Geometry: final body of the model. Coordinates: model frame, mm. A direction names the side the tool comes from. Coordinates: 2 decimals unless noted, no trailing zeros. Loops run counter-clockwise (first coordinate to the right, second up) from the corner with the lowest first, then second, coordinate; pieces in that order, holes last. Notation, with made-up numbers: (-23.75, 81.5) - (-14.75, 81.5) arc R33 ccw to (-14.75, 110.5) - close; hole circle Ø4 at (20.25, 62). An arc over 180 degrees is marked (long way). Return JSON: item names as keys, results as strings.
from build123d import *

# Parameters (mm, degrees)
CROQUIS1_W                 = 70
CROQUIS1_H                 = 70
SALIENTE_EXTRUIR1_DEPTH    = 70
CORTAR_EXTRUIR1_DEPTH      = 122.24355653
CORTAR_EXTRUIR1_DEPTH_BACK = 70
CROQUIS3_W                 = 10
CROQUIS3_H                 = 10
CORTAR_EXTRUIR2_DEPTH      = 70
CORTAR_EXTRUIR3_DEPTH      = 122.24355653
CORTAR_EXTRUIR3_DEPTH_BACK = 122.24355653
CORTAR_EXTRUIR4_DEPTH      = 106.44045021
CORTAR_EXTRUIR4_DEPTH_BACK = 106.44045021
CROQUIS5_W                 = 10
CROQUIS5_H                 = 10


with BuildPart() as part:
    # Croquis1 → Saliente-Extruir1 (new body)
    with BuildSketch(Plane(origin=(0, 0, 0), x_dir=(0, 0, -1), z_dir=(1, 0, 0))):
        with Locations((-35, 35)):
            Rectangle(CROQUIS1_W, CROQUIS1_H)
    extrude(amount=SALIENTE_EXTRUIR1_DEPTH)

    # Croquis2 → Cortar-Extruir1 (cut, two sides: drawn at the far end of the back side and taken through both)
    with BuildSketch(Plane.XY.offset(70).offset(-CORTAR_EXTRUIR1_DEPTH_BACK)):
        Polygon((-82.285109819, 188.585089714), (36.299979895, 70), (70, 36.299979895), (188.585089714, -82.285109819), (425.755269142, 154.885069609), (154.885069609, 425.755269142), align=None)
    extrude(amount=CORTAR_EXTRUIR1_DEPTH + CORTAR_EXTRUIR1_DEPTH_BACK, mode=Mode.SUBTRACT)

    # Croquis3 → Cortar-Extruir2 (cut)
    with BuildSketch(Plane(origin=(70, 0, 0), x_dir=(0, 0, -1), z_dir=(1, 0, 0))):
        with Locations((-15, 5)):
            Rectangle(CROQUIS3_W, CROQUIS3_H)
        with Locations((-55, 5)):
            Rectangle(CROQUIS3_W, CROQUIS3_H)
    extrude(amount=-CORTAR_EXTRUIR2_DEPTH, mode=Mode.SUBTRACT)

    # Croquis4 → Cortar-Extruir3 (cut, two sides: drawn at the far end of the back side and taken through both)
    with BuildSketch(Plane.XY.offset(70).offset(-CORTAR_EXTRUIR3_DEPTH_BACK)):
        Polygon((36.299979895, 237.704642169), (36.299979895, 70), (36.299979895, 60), (46.299979895, 60), (214.004622064, 60), (451.174801491, 297.170179428), (273.470159323, 474.874821596), align=None)
    extrude(amount=CORTAR_EXTRUIR3_DEPTH + CORTAR_EXTRUIR3_DEPTH_BACK, mode=Mode.SUBTRACT)

    # Croquis5 → Cortar-Extruir4 (cut, two sides: drawn at the far end of the back side and taken through both)
    with BuildSketch(Plane(origin=(36.299979895, 0, 0), x_dir=(0, 0, -1), z_dir=(1, 0, 0)).offset(-CORTAR_EXTRUIR4_DEPTH_BACK)):
        with Locations((-35, 65)):
            Rectangle(CROQUIS5_W, CROQUIS5_H)
    extrude(amount=CORTAR_EXTRUIR4_DEPTH + CORTAR_EXTRUIR4_DEPTH_BACK, mode=Mode.SUBTRACT)


solid = part.part
Item 1: Section query D-D, the plane z = 58. Return loops of the section in (x, y).
Worked out:
{"outline": "(0, 10) - (70, 10) - (70, 36.3) - (46.3, 60) - (36.3, 60) - (36.3, 70) - (0, 70) - close"}
Item 2: Section query B-B, the plane z = 21.5. Return loops of the section in (x, y), and give its area (3 significant figures).
Worked out:
{"outline": "(0, 0) - (70, 0) - (70, 36.3) - (46.3, 60) - (36.3, 60) - (36.3, 70) - (0, 70) - close", "area": "4,280 mm^2"}
Item 3: Mould query, pull axis Z, two halves, no side actions, for faces 4 (the face through (18, 65, 30)), 5 (the face through (18, 70, 55)), 6 (the face through (35, 35, 70)). Classes: +Z half, -Z half, draft (parallel to the pull), parting line (faces both ways), or undercut.
Worked out:
{"face 4": "undercut", "face 5": "draft", "face 6": "+Z half"}
Item 4: Section query C-C, the plane y = 54. Return loops of the section in (x, z), and give its area (3 significant figures).
Worked out:
{"outline": "(0, 0) - (52.3, 0) - (52.3, 70) - (0, 70) - close", "area": "3,660 mm^2"}
Item 5: Ray query, probe 1 along Z at (x, y) = (6, 3); probe 2 along Z at (x, y) = (10.5, 64.5); probe 3 along X at (y, z) = (64.5, 45.5). Return the intervals inside material, ascending. Write a range as from..to.
Worked out:
{"probe 1": "0..10, 20..50, 60..70", "probe 2": "0..30, 40..70", "probe 3": "0..36.3"}
Item 6: First-contact query: pin 1 Ø5 at (x, z) = (46.5, 14.5) entering from -Y; pin 2 Ø5 at (y, z) = (65, 56) entering from +X. Flat tips, straight axial feed; report the tip coordinate or a pass-through.
Worked out:
{"pin 1": "y = 10", "pin 2": "x = 36.3"}
Item 7: Section query A-A, the plane x = 39.5. Return loops of the section in (y, z), and give its area (3 significant figures).
Worked out:
{"outline": "(0, 0) - (60, 0) - (60, 70) - (0, 70) - (0, 60) - (10, 60) - (10, 50) - (0, 50) - (0, 20) - (10, 20) - (10, 10) - (0, 10) - close", "area": "4,000 mm^2"}
Item 8: Reachability of faces 1 (the face through (18, 65, 40)), 2 (the face through (36.3, 65, 55)), 3 (the face through (35, 5, 10)) from +Z, -Z, +X, -X, +Y, -Y: full face, straight path, thin tool, end or side. Return the list, or none.
Worked out:
{"face 1": "+X, -X, +Y", "face 2": "+Z, -Z, +X, +Y", "face 3": "+X, -X, -Y"}
